Build history of the part. All positions in model axes, mm. A direction names the side the tool comes from. Round coordinates to 2 decimals unless told otherwise and drop trailing zeros. Write each loop counter-clockwise with the first axis right and the second up, starting at its lowest first coordinate (ties: lowest second). Pieces come first, ordered by that corner, then holes.
from build123d import *

# Parameters (mm, degrees)
ESQUISSE1_R        = 4
ESQUISSE1_R_2      = 3.5
BOSS_EXTRU_1_DEPTH = 1.5
ESQUISSE2_R        = 4.6
ESQUISSE2_R_2      = 4
BOSS_EXTRU_2_DEPTH = 0.5


with BuildPart() as part:
    # Esquisse1 → Boss.-Extru.1 (new, symmetric)
    with BuildSketch(Plane.XY):
        Circle(ESQUISSE1_R)
        Circle(ESQUISSE1_R_2, mode=Mode.SUBTRACT)
    extrude(amount=BOSS_EXTRU_1_DEPTH, both=True)

    # Esquisse2 → Boss.-Extru.2 (add)
    with BuildSketch(Plane.XY.offset(1.5)):
        Circle(ESQUISSE2_R)
        Circle(ESQUISSE2_R_2, mode=Mode.SUBTRACT)
    extrude(amount=-BOSS_EXTRU_2_DEPTH)

    # Esquisse3 → Enlèvement de matière-Révolution1 (revolve, cut)
    with BuildSketch(Plane(origin=(0, 0, 0), x_dir=(1, 0, 0), z_dir=(0, 1, 0)), mode=Mode.PRIVATE) as enl_vement_de_mati_re_r_volution1_sk:
        with BuildLine():
            Line((-3.5, -0.559016994), (-3.5, 0.559016994))
            ThreePointArc((-3.5, 0.559016994), (-3.75, 0), (-3.5, -0.559016994))
        make_face()
    revolve(enl_vement_de_mati_re_r_volution1_sk.sketch.rotate(Axis((0, 0, 1.5), (0, 0, -1)), 180), axis=Axis((0, 0, 1.5), (0, 0, -1)), mode=Mode.SUBTRACT)


solid = part.part
1) Mould opens along Y. For faces 1 (the cylindrical face through (3.233, -1.341, -1.036)), 2 (the flat face through (-2.41, 2.75, 1.5)), 3 (the cylindrical face through (-0.867, -3.905, -0.232)) say: released by +Y, released by -Y, zero draft, split by the parting line, or undercut.
Results:
face 1: undercut
face 2: zero draft
face 3: split by the parting line
2) Which spindle directions (+Z, -Z, +X, -X, +Y, -Y) get a long thin tool onto all of the face, cutting with end or side? Do faces 4 (the cylindrical face through (-3.65, -2.8, 1.25)), 5 (the flat face through (-1.7, 3.8, 1)). Say none if no direction does.
Results:
face 4: +Z, -Z
face 5: -Z
3) Slice it at C-C (z = -0.9). Write the cut outline in (x, y).
Results:
outline: circle Ø8 at (0, 0); hole circle Ø7 at (0, 0)
4) Slice it at D-D (z = 0.1). Write the cut outline in (x, y).
Results:
outline: circle Ø8 at (0, 0); hole circle Ø7.49 at (0, 0)
5) Wall check: L1, parallel to Y at x = 0, z = 1.2; L2, parallel to Z at x = 2.5, y = 3.5; L3, parallel to Y at x = -0.25, z = 0.5. Give the ranges that are in metal, low to high.
Results:
L1: y = -4.6 to -3.5, 3.5 to 4.6
L2: z = 1 to 1.5
L3: y = -3.99 to -3.55, 3.55 to 3.99
6) Pin check, flat tips, straight feed: pin 1 Ø1 at (y, z) = (2, 0) entering from +X; pin 2 Ø1 at (y, z) = (-1, 0) entering from -X. Stop position of each tip, or through.
Results:
pin 1: stops at x = 3.71
pin 2: stops at x = -3.97
7) Slice it at A-A (x = 0). Write the cut outline in (y, z), plus the area to 3 significant figures.
Results:
outline: (-4.6, 1) - (-4, 1) - (-4, -1.5) - (-3.5, -1.5) - (-3.5, -0.56) arc R0.75 cw to (-3.5, 0.56) - (-3.5, 1.5) - (-4.6, 1.5) - close; (3.5, -1.5) - (4, -1.5) - (4, 1) - (4.6, 1) - (4.6, 1.5) - (3.5, 1.5) - (3.5, 0.56) arc R0.75 cw to (3.5, -0.56) - close
area: 3.21 mm2
